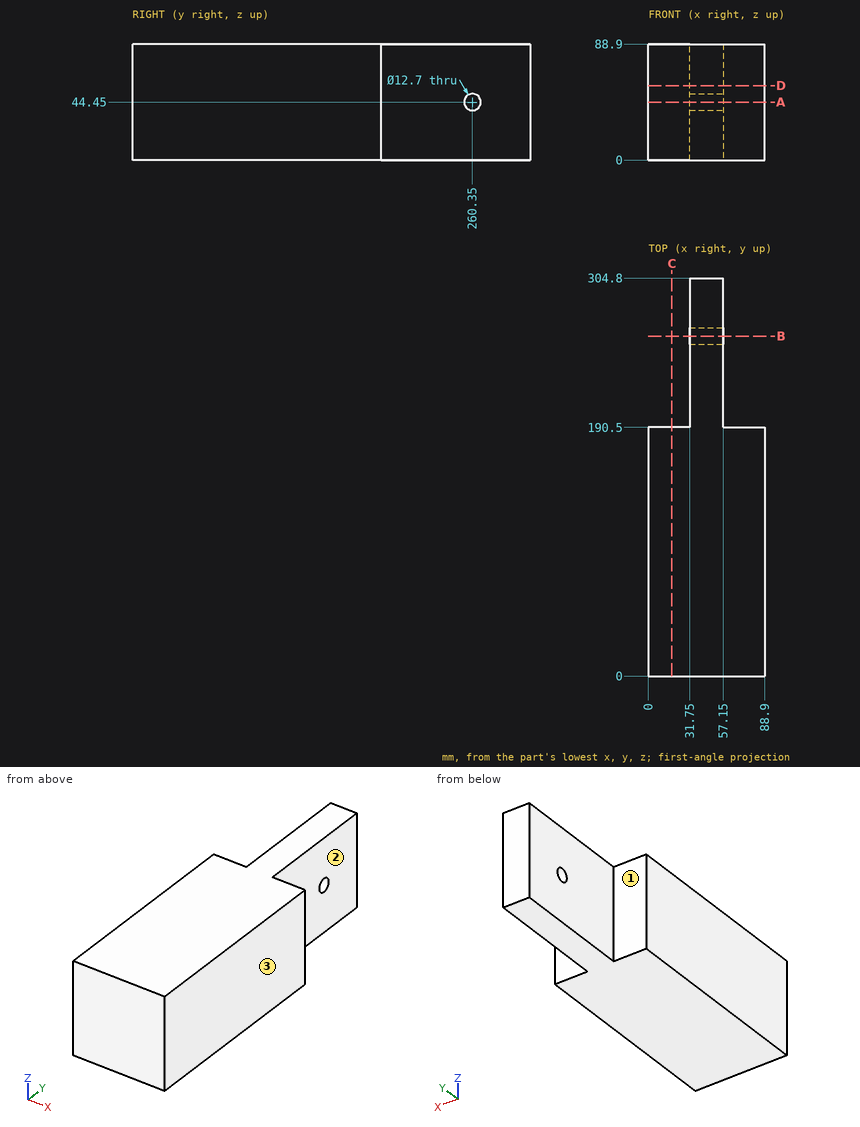
Verification items for this drawing (mm, ordinates from the low corner). A direction names the side the tool comes from. Coordinates: 2 decimals unless noted, no trailing zeros. Loops run counter-clockwise (first coordinate to the right, second up) from the corner with the lowest first, then second, coordinate; pieces in that order, holes last. Notation, with made-up numbers: (-21.5, 34.25) - (0.5, 34.25) arc R19 cw to (0.5, 67.25) - close; hole circle Ø10 at (87, -18.75). An arc over 180 degrees is marked (long way). Use one line per item in the form item = value. Start each with the question number.
Item 1: Section check C-C, the plane x = 18. Enter the section's corners in (y, z).
Item 2: Tool access check on the marked faces 1, 2 and 3. Record the directions out of +Z, -Z, +X, -X, +Y, -Y that give a thin tool (end or side, any length) a straight path to the whole face; none if there is none.
Item 3: Section check D-D, the plane z = 57. Enter the section's corners in (x, y).
Item 4: Thickness scan on probe 1 along Z at (x, y) = (51.75, 260.35); probe 2 along Y at (x, z) = (50, 44); probe 3 along Y at (x, z) = (16, 19). Record the ranges inside material, lowest first.
Item 5: Gauge pin test, flat ends, axial feed: pin 1 (10 mm diameter, centred on y = 262, z = 24.5, fed in from +X); pin 2 (8 mm diameter, centred on x = 21.5, z = 35, fed in from +Y); pin 3 (16.5 mm diameter, centred on y = 260.35, z = 44.45, fed in from -X). Record the tip position at first contact, or that the pin passes through.
Item 6: Section check A-A, the plane z = 44.45. Enter the section's corners in (x, y), and give its area (3 significant figures).
Item 7: Section check B-B, the plane y = 260.35. Enter the section's corners in (x, z), and give its area (3 significant figures).
Computed:
q1.outline = (0, 0) - (190.5, 0) - (190.5, 88.9) - (0, 88.9) - close
q2.face_1 = +Z, -Z, -X, +Y
q2.face_2 = +Z, -Z, +X, +Y
q2.face_3 = +Z, -Z, +X, +Y, -Y
q3.outline = (0, 0) - (88.9, 0) - (88.9, 190.5) - (57.15, 190.5) - (57.15, 304.8) - (31.75, 304.8) - (31.75, 190.5) - (0, 190.5) - close
q4.probe_1 = 0 to 38.1, 50.8 to 88.9
q4.probe_2 = 0 to 254.02, 266.68 to 304.8
q4.probe_3 = 0 to 190.5
q5.pin_1 = 57.15
q5.pin_2 = 190.5
q5.pin_3 = 31.75
q6.outline = (0, 0) - (88.9, 0) - (88.9, 190.5) - (57.15, 190.5) - (57.15, 254) - (31.75, 254) - (31.75, 190.5) - (0, 190.5) - close; (31.75, 266.7) - (57.15, 266.7) - (57.15, 304.8) - (31.75, 304.8) - close
q6.area = 19,500 mm2
q7.outline = (31.75, 0) - (57.15, 0) - (57.15, 38.1) - (31.75, 38.1) - close; (31.75, 50.8) - (57.15, 50.8) - (57.15, 88.9) - (31.75, 88.9) - close
q7.area = 1,940 mm2
